Verification items for the finished model (mm, model axes). A direction names the side the tool comes from. Round coordinates to 2 decimals unless told otherwise and drop trailing zeros. Loops run counter-clockwise (first coordinate to the right, second up) from the corner with the lowest first, then second, coordinate; pieces in that order, holes last. Notation, with made-up numbers: M 19,59.25 L 37,59.25 A9 cw 37,68.25 Z; hole C -22.5,2 d5. An arc over 180 degrees is marked long. Answer as CSV lines item,"result".
Autodesk Inventor part; units mm, degrees
ref_plane "РабПлоскость1" through (-13, -24, -6) normal (0, 0, -1) x (0, 1, 0)
ref_plane "РабПлоскость3" through (-7, 4, -6) normal (-1, 0, 0) x (0, 0, 1)
ref_plane "РабПлоскость6" through (-13, -28.5514, -58.6393) normal (1, 0, 0) x (0, 1, 0)
sketch "Эскиз1" plane through (0, 0, 0) normal (0, 0, 1) x (1, 0, 0)
  line L0 (-10, 17) -> (-7, 17)
  line L1 (-10, 4) -> (-10, 17)
  line L2 (-7, 4) -> (-10, 4)
  line L3 (-7, 17) -> (-7, 4)
  line L4 (-9.9, 4.1) -> (-9.9, 16.9)
  line L5 (-9.9, 16.9) -> (-7.1, 16.9)
  line L6 (-7.1, 16.9) -> (-7.1, 4.1)
  line L7 (-7.1, 4.1) -> (-9.9, 4.1)
  point P0 (0, 0)
  dimension "d22" = 0.1
ref_plane "РабПлоскость1" through (-13, -24, -6) normal (0, 0, -1) x (0, 1, 0)
extrude "Выдавливание1" add sketch "Эскиз1" against normal up to surface (6 mm away) contours L4 L5 L6 L7
ref_plane "РабПлоскость2" through (-13, 2.5481, 2.5558) normal (1, 0, 0) x (0, 1, 0)
sketch "Эскиз3" plane through (-13, 2.5481, 2.5558) normal (1, 0, 0) x (0, 1, 0)
  line L0 (29.663, -39.7893) -> (-15.8657, 56.6115)
  line L1 (1.4519, -2.5558) -> (14.4519, -2.5558)
  circle A0 centre (3.4507, 4.8159) radius 1.5
  circle A1 centre (-0.8198, 13.8581) radius 1.5
  arc A2 (1.3781, 25.1262) -> (1.4519, -2.5558) centre (15.5518, 11.3229) ccw
  line L2 (31.6038, -38.8726) -> (-13.9249, 57.5281)
  point P0 (-2.5481, -2.5558)
  point P1 (-0.157, 23.3504)
  point P2 (12.0781, -2.5558)
ref_plane "РабПлоскость3" through (-7, 4, -6) normal (-1, 0, 0) x (0, 0, 1)
extrude "Выдавливание3" add sketch "Эскиз3" along normal up to surface (6 mm away)
ref_plane "РабПлоскость5" through (-7, 4.2958, -6) normal (1, 0, 0) x (0, 0, -1)
sketch "Эскиз5" plane through (-7, 4.2958, -6) normal (1, 0, 0) x (0, 0, -1)
  spline S0 degree 2 poles (-13.3717, 3.2031) (-15.9697, 3.2031) (-14.6707, 0.9531) (-13.3717, -1.2969) (-12.0726, 0.9531) (-10.7736, 3.2031) (-13.3717, 3.2031) knots 0 0 0 0.333333 0.333333 0.666667 0.666667 1 1 1 weights 1 0.5 1 0.5 1 0.5 1
  circle A0 centre (-13.3717, 1.7031) radius 3
  circle A1 centre (-13.3717, 1.7031) radius 1.5
  circle A2 centre (-13.3717, 1.7031) radius 1.5
  point P0 (-6, -4.2958)
  point P1 (-23.7703, -3.2081)
  point P2 (-23.7703, -3.2081)
  dimension "d12" = 6
extrude "Выдавливание5" cut sketch "Эскиз5" against normal blind 2.5
ref_plane "РабПлоскость4" through (-7, 4.2958, -6) normal (1, 0, 0) x (0, 0, -1)
sketch "Эскиз6" plane through (-7, 4.2958, -6) normal (1, 0, 0) x (0, 0, -1)
  spline S0 degree 2 poles (-22.4139, -1.0675) (-25.012, -1.0675) (-23.713, -3.3175) (-22.4139, -5.5675) (-21.1149, -3.3175) (-19.8159, -1.0675) (-22.4139, -1.0675) knots 0 0 0 0.333333 0.333333 0.666667 0.666667 1 1 1 weights 1 0.5 1 0.5 1 0.5 1
  circle A0 centre (-22.4139, -2.5675) radius 1.5
  circle A1 centre (-22.4139, -2.5675) radius 3
  point P0 (-6, -4.2958)
  dimension "d16" = 6
extrude "Выдавливание6" cut sketch "Эскиз6" against normal blind 4
sketch "Эскиз7" plane through (-7.1, 4, -6) normal (1, 0, 0) x (0, 0, -1)
  line L0 (-6, 13) -> (0, 13)
  line L1 (-6, 13) -> (-33.682, -0.0738)
  line L2 (-33.682, -0.0738) -> (-11.0375, 13)
  line L3 (-6, 13) -> (0, 13)
  line L4 (-6, 13) -> (-11.0375, 13)
  point P0 (-6, -4)
  dimension "d19" = 30
ref_plane "РабПлоскость6" through (-13, -28.5514, -58.6393) normal (1, 0, 0) x (0, 1, 0)
extrude "Выдавливание7" add sketch "Эскиз7" against normal up to surface (5.9 mm away)
properties part number "ЛЦМК.30000.10.00.04  Переходник"
1) Draft check along Y on faces 1 (the flat face through (-10, 17, 2)), 2 (the cylindrical face through (-8.23, 6.9, 4.51)), 3 (the flat face through (-11, 10, 0)), 4 (the flat face through (-11, 1, 18)). Enter one of: +Y half, -Y half, draft (parallel to the pull), parting line (faces both ways), or undercut.
Here are the results:
face 1,"+Y half"
face 2,"undercut"
face 3,"draft"
face 4,"undercut"
2) Section check C-C (x = -8). Record the cut outline in (y, z), plus the area to 3 significant figures.
Here are the results:
outline,"M 3.93,27.68 A19.78 ccw 4,0 L 4.1,0 L 4.1,-6 L 16.9,-6 L 16.9,0 L 17,0 L 17,5.04 Z; hole C 1.73,16.41 d6; hole C 6,7.37 d6"
area,"341 mm^2"
3) Section check A-A (z = 7). Record the cut outline in (x, y).
Here are the results:
outline,"M -13,-0.45 L -7,-0.45 L -7,3.02 L -9.5,3.02 L -9.5,4.55 L -13,4.55 Z; M -13,7.45 L -9.5,7.45 L -9.5,8.98 L -7,8.98 L -7,13.69 L -7.1,13.69 L -7.1,15.87 L -13,15.87 Z"
4) Material ranges on probe 1 along Z at (x, y) = (-7.5, 3.25); probe 2 along Y at (x, z) = (-8.25, 5.5); probe 3 along Y at (x, z) = (-7.5, 16), recorded low to high.
Here are the results:
probe 1,"z = 0.81 to 6.17, 8.57 to 13.83, 19 to 26.95"
probe 2,"y = 0.18 to 3.65, 8.34 to 16.73"
probe 3,"y = -1.57 to -1.24, 4.7 to 10.67"
5) Set-up check for faces 5 (the flat face through (-9.9, 10, -3)), 6 (the flat face through (-8, 4.1, -3)), 7 (the flat face through (-9.5, 5, 9)): record each of +Z, -Z, +X, -X, +Y, -Y from which the full face is reachable in a straight line by a thin tool's end or side.
Here are the results:
face 5,"-Z, -X, +Y, -Y"
face 6,"-Z, +X, -X, -Y"
face 7,"+X"
6) Go/stop test with flat-tipped pins: pin 1 (5 mm diameter, centred on y = 12.5, z = -4, fed in from +X); pin 2 (3.5 mm diameter, centred on y = 6, z = 7.37, fed in from +X); pin 3 (1.4 mm diameter, centred on x = -9, z = -3.5, fed in from -Y); pin 4 (1.8 mm diameter, centred on y = 1.73, z = 16.41, fed in from +X). Record where each tip stops, or that it passes through.
Here are the results:
pin 1,"stops at x = -7.1"
pin 2,"stops at x = -9.5"
pin 3,"stops at y = 4.1"
pin 4,"passes through"
7) Section check D-D (z = 14). Record the cut outline in (x, y).
Here are the results:
outline,"M -13,-1.68 L -7,-1.68 L -7,-0.05 L -11,-0.05 L -11,3.51 L -7,3.51 L -7,10.39 L -7.1,10.39 L -7.1,11.83 L -13,11.83 Z"
8) Section check B-B (y = 14.25). Record the cut outline in (x, z), plus the area to 3 significant figures.
Here are the results:
outline,"M -13,0 L -9.9,0 L -9.9,-6 L -7.1,-6 L -7.1,0 L -7,0 L -7,5.82 L -7.1,5.82 L -7.1,9.8 L -13,9.8 Z"
area,"75.2 mm^2"
